Read the model definition and answer for the solid it produces. Units are mm, in the model's axes. Give positions to 0.01 mm unless a question says otherwise; leave off trailing zeros. Loops run counter-clockwise (first coordinate to the right, second up) from the corner with the lowest first, then second, coordinate; pieces in that order, holes last. Notation, with made-up numbers: (40, 65.25) - (86, 65.25) arc R11 ccw to (86, 72.25) - close; hole circle Ø1 at (-33.5, -9). An arc over 180 degrees is marked (long way). Write item = value, one per line. Start each with the question number.
from build123d import *

# Parameters (mm, degrees)
SKETCH1_W                                = 152.4
SKETCH1_H                                = 239.776
BOSS_EXTRUDE1_DEPTH                      = 5.588
CUT_EXTRUDE6_DEPTH                       = 432.430054712
MIRROR1_AT_THE_SECOND_PLANE_COPY_1_DEPTH = 432.430054712
SKETCH8_W                                = 239.776
SKETCH8_H                                = 5.588
BOSS_EXTRUDE2_DEPTH                      = 25.4
CUT_EXTRUDE7_DEPTH                       = 158.247951618
SKETCH10_R                               = 6
CUT_EXTRUDE8_DEPTH                       = 456.882202726


with BuildPart() as part:
    # Sketch1 → Boss-Extrude1 (new body)
    with BuildSketch(Plane(origin=(0, 0, 0), x_dir=(1, 0, 0), z_dir=(0, 1, 0))):
        Rectangle(SKETCH1_W, SKETCH1_H)
    extrude(amount=BOSS_EXTRUDE1_DEPTH)

    # Sketch7 → Cut-Extrude6 (cut, through all)
    with BuildSketch(Plane(origin=(-338.200209725, 5.588, 0), x_dir=(1, 0, 0), z_dir=(0, 1, 0))):
        with BuildLine():
            Line((268.819954903, 97.377738503), (268.819954903, 110.077738503))
            ThreePointArc((268.819954903, 110.077738503), (271.469954903, 112.727738503), (274.119954903, 110.077738503))
            Line((274.119954903, 110.077738503), (274.119954903, 97.377738503))
            ThreePointArc((274.119954903, 97.377738503), (271.469954903, 94.727738503), (268.819954903, 97.377738503))
        make_face()
    cut_extrude6 = extrude(amount=-CUT_EXTRUDE6_DEPTH, mode=Mode.SUBTRACT)

    # Mirror1: Cut-Extrude6 across plane
    add(cut_extrude6.mirror(Plane.XY), mode=Mode.SUBTRACT)

    # Mirror1 at the second plane: Cut-Extrude6 across plane
    add(cut_extrude6.mirror(Plane(origin=(0, 0, 0), x_dir=(0, 0, 1), z_dir=(1, 0, 0))), mode=Mode.SUBTRACT)

    # Mirror1 at the second plane copy 1 sketc → Mirror1 at the second plane copy 1 (cut, through all)
    with BuildSketch(Plane(origin=(338.200209725, 5.588, 0), x_dir=(-1, 0, 0), z_dir=(0, 1, 0))):
        with BuildLine():
            Line((268.819954903, 97.377738503), (268.819954903, 110.077738503))
            ThreePointArc((268.819954903, 110.077738503), (271.469954903, 112.727738503), (274.119954903, 110.077738503))
            Line((274.119954903, 110.077738503), (274.119954903, 97.377738503))
            ThreePointArc((274.119954903, 97.377738503), (271.469954903, 94.727738503), (268.819954903, 97.377738503))
        make_face()
    extrude(amount=-MIRROR1_AT_THE_SECOND_PLANE_COPY_1_DEPTH, mode=Mode.SUBTRACT)

    # Sketch8 → Boss-Extrude2 (add)
    with BuildSketch(Plane.ZY.offset(76.2)):
        with Locations((0, 2.794)):
            Rectangle(SKETCH8_W, SKETCH8_H)
    boss_extrude2 = extrude(amount=BOSS_EXTRUDE2_DEPTH)

    # Sketch9 → Cut-Extrude7 (cut, through all)
    with BuildSketch(Plane(origin=(0, 5.588, 0), x_dir=(1, 0, 0), z_dir=(0, 1, 0))):
        with BuildLine():
            Line((-69.380254823, 110.077738503), (-69.380254823, 97.377738503))
            ThreePointArc((-69.380254823, 97.377738503), (-66.730254823, 94.727738503), (-64.080254823, 97.377738503))
            Line((-64.080254823, 97.377738503), (-64.080254823, 110.077738503))
            ThreePointArc((-64.080254823, 110.077738503), (-66.730254823, 112.727738503), (-69.380254823, 110.077738503))
        make_face()
        with BuildLine():
            Line((-88.319745177, 97.377738503), (-88.319745177, 110.077738503))
            ThreePointArc((-88.319745177, 110.077738503), (-85.669745177, 112.727738503), (-83.019745177, 110.077738503))
            Line((-83.019745177, 110.077738503), (-83.019745177, 97.377738503))
            ThreePointArc((-83.019745177, 97.377738503), (-85.669745177, 94.727738503), (-88.319745177, 97.377738503))
        make_face()
        with BuildLine():
            Line((-88.319745177, -97.377738503), (-88.319745177, -110.077738503))
            ThreePointArc((-88.319745177, -110.077738503), (-85.669745177, -112.727738503), (-83.019745177, -110.077738503))
            Line((-83.019745177, -110.077738503), (-83.019745177, -97.377738503))
            ThreePointArc((-83.019745177, -97.377738503), (-85.669745177, -94.727738503), (-88.319745177, -97.377738503))
        make_face()
    cut_extrude7 = extrude(amount=-CUT_EXTRUDE7_DEPTH, mode=Mode.SUBTRACT)

    # Mirror2: Boss-Extrude2, Cut-Extrude7 across plane
    add(boss_extrude2.mirror(Plane(origin=(0, 0, 0), x_dir=(0, 0, 1), z_dir=(1, 0, 0))))
    add(cut_extrude7.mirror(Plane(origin=(0, 0, 0), x_dir=(0, 0, 1), z_dir=(1, 0, 0))), mode=Mode.SUBTRACT)

    # Sketch10 → Cut-Extrude8 (cut, through all)
    with BuildSketch(Plane(origin=(-338.200209725, 5.588, 0), x_dir=(1, 0, 0), z_dir=(0, 1, 0))):
        with Locations(Location((269.176273717, -20.727348554, 0), (0, 0, 270))):
            Circle(SKETCH10_R)
    cut_extrude8 = extrude(amount=-CUT_EXTRUDE8_DEPTH, mode=Mode.SUBTRACT)

    # Mirror3: Cut-Extrude8 across plane
    add(cut_extrude8.mirror(Plane(origin=(0, 0, 0), x_dir=(0, 0, 1), z_dir=(1, 0, 0))), mode=Mode.SUBTRACT)


solid = part.part
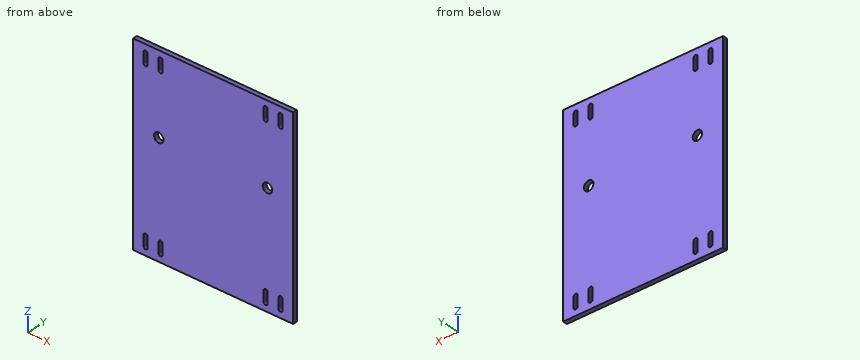
1. Consider line 1 along X through (y, z) = (4, 106); line 2 along Z through (x, y) = (86.5, 0.7); line 3 along X through (y, z) = (1.55, 25). Determine where each line is inside the solid, lowest interval first. Write a range as [from, to].
2. A cutting plane is placed at A-A on z = 18.5. Give the vertices of the cut face in (x, y).
3. A cutting plane is placed at B-B on y = 3.3. Give the number of separate pieces and of enclosed holes in the cut face, and give its area (3 significant figures).
Reply:
q1.line_1 = [-101.6, -88.32], [-83.02, -69.38], [-64.08, 64.08], [69.38, 83.02], [88.32, 101.6]
q1.line_2 = [-119.89, -112.59], [-94.86, 94.86], [112.59, 119.89]
q1.line_3 = [-101.6, -73.24], [-64.81, 64.81], [73.24, 101.6]
q2.outline = (-101.6, 0) - (-74.6, 0) - (-74.6, 5.59) - (-101.6, 5.59) - close; (-63.45, 0) - (63.45, 0) - (63.45, 5.59) - (-63.45, 5.59) - close; (74.6, 0) - (101.6, 0) - (101.6, 5.59) - (74.6, 5.59) - close
q3.separate_pieces = 1
q3.enclosed_holes = 10
q3.area = 47,800 mm^2
